Autodesk Inventor part; units mm, degrees
ref_plane "YZ Plane" through (0, 0, 0) normal (1, 0, 0) x (0, 1, 0)
ref_plane "XZ Plane" through (0, 0, 0) normal (0, 1, 0) x (-1, 0, 0)
ref_plane "XY Plane" through (0, 0, 0) normal (0, 0, 1) x (1, 0, 0)
sketch "Эскиз1" plane through (0, 0, 0) normal (0, 0, 1) x (1, 0, 0)
  line L0 (-125, -45) -> (125, -45)
  line L1 (125, -45) -> (125, 45)
  line L2 (125, 45) -> (-125, 45)
  line L3 (-125, 45) -> (-125, -45)
  line L4 (-125, -45) -> (125, 45) construction
  line L5 (125, -45) -> (-125, 45) construction
  line L6 (32.5, -80) -> (-32.5, -80)
  line L7 (-32.5, -80) -> (-32.5, 80)
  line L8 (-32.5, 80) -> (32.5, 80)
  line L9 (32.5, 80) -> (32.5, -80)
  line L10 (32.5, -80) -> (-32.5, 80) construction
  line L11 (-32.5, -80) -> (32.5, 80) construction
  point P0 (0, 0)
  dimension "d0" = 250
  dimension "d1" = 90
  dimension "d2" = 65
  dimension "d3" = 160
extrude "Выдавливание1" add sketch "Эскиз1" along normal blind 10
sketch "Эскиз2" plane through (0, 0, 10) normal (0, 0, 1) x (1, 0, 0)
  line L0 (16, 68) -> (-16, 68) construction
  line L1 (-16, 68) -> (-16, 80) construction
  line L2 (-16, 80) -> (16, 80) construction
  line L3 (16, 80) -> (16, 68) construction
  line L4 (16, 68) -> (-16, 80) construction
  line L5 (-16, 68) -> (16, 80) construction
  line L6 (0, 0) -> (16, 0) construction
  line L7 (16, -68) -> (-16, -68) construction
  line L8 (-16, -68) -> (-16, -80) construction
  line L9 (-16, -80) -> (16, -80) construction
  line L10 (16, -80) -> (16, -68) construction
  line L11 (16, -68) -> (-16, -80) construction
  line L12 (-16, -68) -> (16, -80) construction
  circle A0 centre (-16, 68) radius 2
  circle A1 centre (16, 68) radius 2
  circle A2 centre (-16, -68) radius 2
  circle A3 centre (16, -68) radius 2
  point P0 (0, 74)
  point P1 (-32.5, 80)
  point P2 (0, 74)
  point P3 (0, 74)
  point P4 (0, -74)
  point P5 (-32.5, -80)
  point P6 (0, -74)
  point P7 (0, -74)
  dimension "d6" = 32
  dimension "d7" = 12
  dimension "d8" = 4
  dimension "d9" = 4
  dimension "d10" = 4
  dimension "d11" = 4
extrude "Выдавливание2" cut sketch "Эскиз2" against normal blind 10
sketch "Эскиз3" plane through (0, 0, 10) normal (0, 0, 1) x (1, 0, 0)
  line L0 (100, -40) -> (-60, -40) construction
  line L1 (-60, -40) -> (-60, 40) construction
  line L2 (-60, 40) -> (100, 40) construction
  line L3 (100, 40) -> (100, -40) construction
  line L4 (100, -40) -> (-60, 40) construction
  line L5 (-60, -40) -> (100, 40) construction
  line L6 (125, -45) -> (125, 45) construction
  circle A0 centre (100, 40) radius 2
  circle A1 centre (100, -40) radius 2
  circle A2 centre (-60, -40) radius 2
  circle A3 centre (-60, 40) radius 2
  point P0 (0, 0)
  point P1 (20, 0)
  point P2 (20, 0)
  dimension "d14" = 160
  dimension "d15" = 80
  dimension "d16" = 25
  dimension "d17" = 4
  dimension "d18" = 4
  dimension "d19" = 4
  dimension "d20" = 4
extrude "Выдавливание3" cut sketch "Эскиз3" against normal blind 10
sketch "Эскиз4" plane through (0, 0, 10) normal (0, 0, 1) x (1, 0, 0)
  line L0 (-113, -12.5) -> (-73, -12.5) construction
  line L1 (-73, -12.5) -> (-73, 12.5) construction
  line L2 (-73, 12.5) -> (-113, 12.5) construction
  line L3 (-113, 12.5) -> (-113, -12.5) construction
  line L4 (-113, -12.5) -> (-73, 12.5) construction
  line L5 (-73, -12.5) -> (-113, 12.5) construction
  line L6 (-125, 45) -> (-125, -45) construction
  circle A0 centre (-113, 12.5) radius 1.5
  circle A1 centre (-73, 12.5) radius 1.5
  circle A2 centre (-73, -12.5) radius 1.5
  circle A3 centre (-113, -12.5) radius 1.5
  point P0 (0, 0)
  point P1 (-93, 0)
  point P2 (-93, 0)
  dimension "d23" = 40
  dimension "d24" = 25
  dimension "d25" = 12
  dimension "d26" = 3
  dimension "d27" = 3
  dimension "d28" = 3
  dimension "d29" = 3
extrude "Выдавливание4" cut sketch "Эскиз4" against normal blind 10
sketch "Эскиз5" plane through (0, 0, 10) normal (0, 0, 1) x (1, 0, 0)
  line L0 (-51, -23.5) -> (-61, -23.5)
  line L1 (-61, -23.5) -> (-61, 23.5)
  line L2 (-61, 23.5) -> (-51, 23.5)
  line L3 (-51, 23.5) -> (-51, -23.5)
  line L4 (-51, -23.5) -> (-61, 23.5) construction
  line L5 (-61, -23.5) -> (-51, 23.5) construction
  circle A0 centre (-73, 12.5) radius 1.5
  point P0 (0, 0)
  point P1 (-56, 0)
  point P2 (-56, 0)
  dimension "d32" = 10
  dimension "d33" = 47
  dimension "d34" = 12
extrude "Выдавливание5" cut sketch "Эскиз5" against normal blind 10 contours L0 L1 L2 L3
sketch "Эскиз6" plane through (0, 0, 10) normal (0, 0, 1) x (1, 0, 0)
  line L0 (-18, -25) -> (-48, -25) construction
  line L1 (-48, -25) -> (-48, 25) construction
  line L2 (-48, 25) -> (-18, 25) construction
  line L3 (-18, 25) -> (-18, -25) construction
  line L4 (-18, -25) -> (-48, 25) construction
  line L5 (-48, -25) -> (-18, 25) construction
  line L6 (-51, 23.5) -> (-51, -23.5) construction
  circle A0 centre (-48, 25) radius 1.5
  circle A1 centre (-18, 25) radius 1.5
  circle A2 centre (-18, -25) radius 1.5
  circle A3 centre (-48, -25) radius 1.5
  point P0 (0, 0)
  point P1 (-33, 0)
  point P2 (-33, 0)
  dimension "d37" = 30
  dimension "d38" = 50
  dimension "d39" = 3
  dimension "d40" = 3
  dimension "d41" = 3
  dimension "d42" = 3
  dimension "d43" = 3
extrude "Выдавливание6" cut sketch "Эскиз6" against normal blind 10
sketch "Эскиз7" plane through (0, 0, 10) normal (0, 0, 1) x (1, 0, 0)
  circle A0 centre (-10, -18.5758) radius 1.375
  circle A1 centre (39, -18.5758) radius 1.375
  circle A2 centre (39, 39.4242) radius 1.375
  circle A3 centre (-10, 39.4242) radius 1.375
  point P0 (0, 0)
extrude "Выдавливание7" cut sketch "Эскиз7" against normal blind 10
properties part number "Основная пластина платформы"
The listing builds one solid part. Answer for the finished solid, in the listing's coordinates (mm). A direction names the side the tool comes from. Give positions to 0.01 mm unless a question says otherwise; leave off trailing zeros. Loops run counter-clockwise (first coordinate to the right, second up) from the corner with the lowest first, then second, coordinate; pieces in that order, holes last. Notation, with made-up numbers: (41, 21.25) - (60, 21.25) arc R18 cw to (60, 49.25) - close; hole circle Ø7 at (-26, 24.5). An arc over 180 degrees is marked (long way). Write each question's results on one line, items separated by ' | '.
1. For a pull along Y with two mould halves and no side action, classify faces 1 (the face through (-32.5, 62, 5)), 2 (the face through (0, 80, 5)), 3 (the face through (-51, 0, 5)) as +Y half, -Y half, draft (parallel to the pull), parting line (faces both ways), or undercut.
Resolved:
face 1: draft | face 2: +Y half | face 3: undercut
2. Find section A-A, the plane y = 17.5. Write down the section's boundary in (x, z).
Resolved:
outline: (-125, 0) - (-61, 0) - (-61, 10) - (-125, 10) - close; (-51, 0) - (125, 0) - (125, 10) - (-51, 10) - close
3. Which of the six approach directions +Z, -Z, +X, -X, +Y, -Y give full straight-line access (tool end or side, diameter ignored) to faces 4 (the face through (32.5, -62, 5)), 5 (the face through (-78, 45, 5)), 6 (the face through (-56, 23.5, 5)), 7 (the face through (-79, -45, 5)), 8 (the face through (79, 45, 5))?
Resolved:
face 4: +Z, -Z, +X, -Y | face 5: +Z, -Z, -X, +Y | face 6: +Z, -Z | face 7: +Z, -Z, -X, -Y | face 8: +Z, -Z, +X, +Y
4. Find section C-C, the plane z = 7.75. Count the separate pieces of the cut face and the enclosed holes in it, then the cut area to 3 significant figures.
Resolved:
separate pieces: 1 | enclosed holes: 21 | area: 26,400 mm^2
5. Consider probe 1 along Y at (x, z) = (-73, 6.75); probe 2 along Y at (x, z) = (-48, 3.25); probe 3 along X at (y, z) = (20, 4). Determine where each line is inside the solid, lowest interval first. Write a range as from..to.
Resolved:
probe 1: y = -45..-14, -11..11, 14..45 | probe 2: y = -45..-26.5, -23.5..23.5, 26.5..45 | probe 3: x = -125..-61, -51..125
6. Find section B-B, the plane x = 106. Write down the section's boundary in (y, z), then the cut area to 3 significant figures.
Resolved:
outline: (-45, 0) - (45, 0) - (45, 10) - (-45, 10) - close | area: 900 mm^2
7. Flat-ended cylindrical pins translate along their axes: P1, Ø5, axis at x = 16, y = -68, coming from the -Z side; P2, Ø5, axis at x = 77.5, z = 5, coming from the -Y side; P3, Ø3, axis at x = -71, z = 4.5, coming from the +Y side; P4, Ø2.5, axis at x = -48, y = 25, coming from the +Z side. Find the tip coordinate at first contact, or state that the pin passes through.
Resolved:
P1: stops at z = 0 | P2: stops at y = -45 | P3: stops at y = 45 | P4: passes through
